Here's how the part is built. I have some questions about the finished solid (model axes, mm). Face numbers are marked on the shaded views. A direction names the side the tool comes from. Give positions to 0.01 mm unless a question says otherwise; leave off trailing zeros. Loops run counter-clockwise (first coordinate to the right, second up) from the corner with the lowest first, then second, coordinate; pieces in that order, holes last. Notation, with made-up numbers: M 42.25,20.5 L 93.25,20.5 A24 ccw 93.25,56.5 Z; hole C 66,50.5 d7. An arc over 180 degrees is marked long. Answer as CSV lines item,"result". Start each with the question number.
Item 1: I want a section at C-C on x = -15. List the corners of the cut face in (y, z) for me.
Item 2: I want a section at D-D on y = 1.5. List the corners of the cut face in (x, z) for me.
Item 3: If I drill on line 1 along Y through (x, z) = (-17, 10.75); line 2 along Z through (x, y) = (-5.5, 17.25); line 3 along Y through (x, z) = (-22, 16.5), over which ranges is the centre line in solid material (lowest first)? Write a range as from..to.
Item 4: I want a section at A-A on x = 11. List the corners of the cut face in (y, z) for me.
Item 5: Will this pin go through, and if not, where does the flat tip stop? P1, Ø3, axis at x = -26, y = 12, coming from the +Z side.
Item 6: If we mould it in two halves opening along Z, with no side actions, what happens to the marked faces 1, 2, 3 and 4? For each: released by +Z, released by -Z, zero draft, split by the parting line, or undercut.
Item 7: For the marked faces 5 and 6, which set-ups out of +Z, -Z, +X, -X, +Y, -Y let a thin tool reach every point of the face, with its end or its side?
Item 8: I want a section at B-B on z = 11. List the corners of the cut face in (x, y) for me, plus the area to 3 significant figures.
from build123d import *

# Parameters (mm, degrees)
F0_W     = 50
F0_H     = 30
F1_DEPTH = 15
F2_T     = -2.5
F3_W     = 50
F3_H     = 30
F3_R     = 4.25
F4_DEPTH = 2.5


with BuildPart() as f1:
    # F0 (on Top) → F1 (new body)
    with BuildSketch(Plane.XY):
        with Locations((-9.941086, 6.442985)):
            Rectangle(F0_W, F0_H)
    extrude(amount=F1_DEPTH)

    # F2
    f2_openings = [f1.faces().sort_by_distance(p)[0] for p in [
        (-9.941086, 6.442985, 15),
    ]]
    offset(amount=F2_T, openings=f2_openings)

    # F3 (on face) → F4 (join)
    with BuildSketch(Plane.XY.offset(15)):
        with Locations((-9.941086, 6.442985)):
            Rectangle(F3_W, F3_H)
        with BuildLine():
            ThreePointArc((-22.246402, -2.057015), (-30.941643, 6.344522), (-22.441086, 14.942985))
            Line((-22.441086, 14.942985), (-12.441086, 14.942985))
            ThreePointArc((-12.441086, 14.942985), (-3.940528, 6.539219), (-12.246402, -2.057015))
            Line((-12.246402, -2.057015), (-22.246402, -2.057015))
        make_face(mode=Mode.SUBTRACT)
        with Locations((4.558914, 6.442985)):
            Circle(F3_R, mode=Mode.SUBTRACT)
    extrude(amount=F4_DEPTH)


solid = f1.part
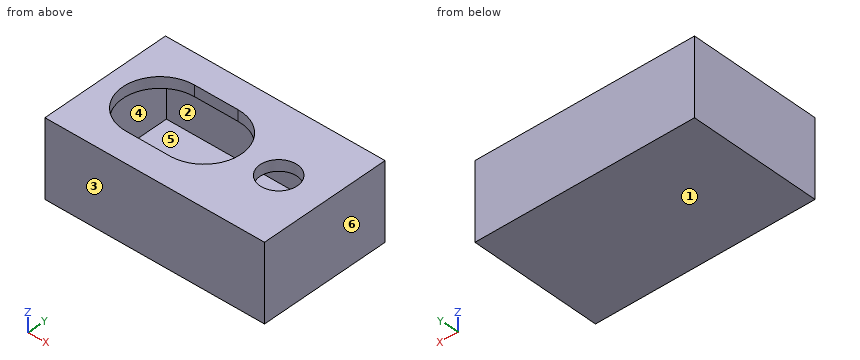
Result:
1,outline,"M -8.56,0 L 21.44,0 L 21.44,17.5 L 14.94,17.5 L 14.94,15 L 18.94,15 L 18.94,2.5 L -6.06,2.5 L -6.06,15 L -2.06,15 L -2.06,17.5 L -8.56,17.5 Z"
2,outline,"M -34.94,0 L 15.06,0 L 15.06,17.5 L -5.52,17.5 L -5.52,15 L 12.56,15 L 12.56,2.5 L -32.44,2.5 L -32.44,15 L -29.36,15 L -29.36,17.5 L -34.94,17.5 Z"
3,line 1,"-8.56..-6.06, 18.94..21.44"
3,line 2,"0..2.5, 15..17.5"
3,line 3,"-8.56..-2.06, 14.94..21.44"
4,outline,"M -8.56,0 L 21.44,0 L 21.44,17.5 L -8.56,17.5 Z; hole M -6.06,2.5 L 18.94,2.5 L 18.94,15 L -6.06,15 Z"
5,P1,"z = 2.5"
6,face 1,"released by -Z"
6,face 2,"undercut"
6,face 3,"zero draft"
6,face 4,"undercut"
7,face 5,"none"
7,face 6,"+Z, -Z, +X, +Y, -Y"
8,outline,"M -34.94,-8.56 L 15.06,-8.56 L 15.06,21.44 L -34.94,21.44 Z; hole M -32.44,-6.06 L 12.56,-6.06 L 12.56,18.94 L -32.44,18.94 Z"
8,area,"375 mm^2"
